Geometry: final body of the model. Coordinates: model frame, mm. Give positions to 0.01 mm unless a question says otherwise; leave off trailing zeros. Order: outer loops, then holes, each group sorted by start corner. A loop starts at its lowest first (then second) coordinate and runs counter-clockwise, first axis right, second up. Notation, with made-up numbers: M 54,88 L 71,88 A19 ccw 71,94 Z; hole C 14.5,-2 d3. An arc over 180 degrees is marked long. Use CSV: the item, a comma, the result in double quotes.
```python
from build123d import *

# Parameters (mm, degrees)
SKETCH1_W           = 224.4
SKETCH1_H           = 224.4
SKETCH1_R           = 1.5
BOSS_EXTRUDE1_DEPTH = 3
FILLET1_R           = 5
SKETCH2_R           = 1
CUT_EXTRUDE1_DEPTH  = 4
SKETCH4_R           = 4.9
CUT_EXTRUDE2_DEPTH  = 4


with BuildPart() as part:
    # Sketch1 → Boss-Extrude1 (new body)
    with BuildSketch(Plane(origin=(0, 0, 0), x_dir=(1, 0, 0), z_dir=(0, 1, 0))):
        with Locations((112.2, 112.2)):
            Rectangle(SKETCH1_W, SKETCH1_H)
        with Locations((213.9, 10.5)):
            Circle(SKETCH1_R, mode=Mode.SUBTRACT)
        with Locations((213.9, 213.9)):
            Circle(SKETCH1_R, mode=Mode.SUBTRACT)
        with Locations((10.5, 10.5)):
            Circle(SKETCH1_R, mode=Mode.SUBTRACT)
        with Locations((10.5, 213.9)):
            Circle(SKETCH1_R, mode=Mode.SUBTRACT)
    extrude(amount=BOSS_EXTRUDE1_DEPTH)

    # Fillet1
    fillet1_edges = [part.edges().sort_by_distance(p)[0] for p in [
        (0, 1.5, -224.4),
        (224.4, 1.5, -224.4),
        (224.4, 1.5, 0),
        (0, 1.5, 0),
    ]]
    fillet(fillet1_edges, radius=FILLET1_R)

    # Sketch2 → Cut-Extrude1 (cut, through all)
    with BuildSketch(Plane(origin=(0, 3, 0), x_dir=(1, 0, 0), z_dir=(0, 1, 0))):
        with Locations((117.180175368, 112.100128542)):
            Circle(SKETCH2_R)
        with Locations((122.180175368, 112.100128542)):
            Circle(SKETCH2_R)
        with Locations((127.180175368, 112.100128542)):
            Circle(SKETCH2_R)
        with Locations((114.680175368, 107.770001523)):
            Circle(SKETCH2_R)
        with Locations((109.680175368, 107.770001523)):
            Circle(SKETCH2_R)
        with Locations((107.180175368, 112.100128542)):
            Circle(SKETCH2_R)
        with Locations((109.680175368, 116.430255561)):
            Circle(SKETCH2_R)
        with Locations((114.680175368, 116.430255561)):
            Circle(SKETCH2_R)
        with Locations((120.840429406, 107.100128542)):
            Circle(SKETCH2_R)
        with Locations((117.180175368, 103.439874505)):
            Circle(SKETCH2_R)
        with Locations((112.180175368, 102.100128542)):
            Circle(SKETCH2_R)
        with Locations((107.180175368, 103.439874505)):
            Circle(SKETCH2_R)
        with Locations((103.51992133, 107.100128542)):
            Circle(SKETCH2_R)
        with Locations((102.180175368, 112.100128542)):
            Circle(SKETCH2_R)
        with Locations((103.51992133, 117.100128542)):
            Circle(SKETCH2_R)
        with Locations((107.180175368, 120.76038258)):
            Circle(SKETCH2_R)
        with Locations((112.180175368, 122.100128542)):
            Circle(SKETCH2_R)
        with Locations((117.180175368, 120.76038258)):
            Circle(SKETCH2_R)
        with Locations((120.840429406, 117.100128542)):
            Circle(SKETCH2_R)
        with Locations((126.669062762, 108.217842866)):
            Circle(SKETCH2_R)
        with Locations((125.170556425, 104.600128542)):
            Circle(SKETCH2_R)
        with Locations((122.786777086, 101.493526825)):
            Circle(SKETCH2_R)
        with Locations((119.680175368, 99.109747486)):
            Circle(SKETCH2_R)
        with Locations((116.062461045, 97.611241148)):
            Circle(SKETCH2_R)
        with Locations((112.180175368, 97.100128542)):
            Circle(SKETCH2_R)
        with Locations((108.297889692, 97.611241148)):
            Circle(SKETCH2_R)
        with Locations((104.680175368, 99.109747486)):
            Circle(SKETCH2_R)
        with Locations((101.57357365, 101.493526825)):
            Circle(SKETCH2_R)
        with Locations((99.189794311, 104.600128542)):
            Circle(SKETCH2_R)
        with Locations((97.691287974, 108.217842866)):
            Circle(SKETCH2_R)
        with Locations((97.180175368, 112.100128542)):
            Circle(SKETCH2_R)
        with Locations((97.691287974, 115.982414219)):
            Circle(SKETCH2_R)
        with Locations((99.189794311, 119.600128542)):
            Circle(SKETCH2_R)
        with Locations((101.57357365, 122.70673026)):
            Circle(SKETCH2_R)
        with Locations((104.680175368, 125.090509599)):
            Circle(SKETCH2_R)
        with Locations((108.297889692, 126.589015937)):
            Circle(SKETCH2_R)
        with Locations((112.180175368, 127.100128542)):
            Circle(SKETCH2_R)
        with Locations((116.062461045, 126.589015937)):
            Circle(SKETCH2_R)
        with Locations((119.680175368, 125.090509599)):
            Circle(SKETCH2_R)
        with Locations((122.786777086, 122.70673026)):
            Circle(SKETCH2_R)
        with Locations((125.170556425, 119.600128542)):
            Circle(SKETCH2_R)
        with Locations((126.669062762, 115.982414219)):
            Circle(SKETCH2_R)
    extrude(amount=-CUT_EXTRUDE1_DEPTH, mode=Mode.SUBTRACT)

    # Sketch4 → Cut-Extrude2 (cut, through all)
    with BuildSketch(Plane(origin=(0, 3, 0), x_dir=(1, 0, 0), z_dir=(0, 1, 0))):
        with Locations((112.2, 157.2)):
            Circle(SKETCH4_R)
        with Locations((157.2, 112.2)):
            Circle(SKETCH4_R)
        with Locations((112.2, 67.2)):
            Circle(SKETCH4_R)
        with Locations((67.2, 112.2)):
            Circle(SKETCH4_R)
    extrude(amount=-CUT_EXTRUDE2_DEPTH, mode=Mode.SUBTRACT)


solid = part.part
```
1. Section A-A, the plane z = -157.2. Return the cut outline in (x, y).
Answer:
outline,"M 0,0 L 107.3,0 L 107.3,3 L 0,3 Z; M 117.1,0 L 224.4,0 L 224.4,3 L 117.1,3 Z"
2. Pull-direction query (X, two-part tool) for faces 1 (the face through (111, 3, -114)), 2 (the face through (1.43, 1.52, -222.9)), 3 (the face through (69.834, 1.521, -116.332)); classes: +X half, -X half, draft (parallel to the pull), parting line (faces both ways), or undercut.
Answer:
face 1,"draft"
face 2,"-X half"
face 3,"undercut"
3. Pin query (flat end, axial travel): pin 1 Ø3 at (x, z) = (117.18, -120.76) entering from -Y. Return the tip coordinate at first contact, or that it passes through.
Answer:
pin 1,"y = 0"
4. Section B-B, the plane x = 66. Return the cut outline in (y, z), plus the area to 3 significant figures.
Answer:
outline,"M 0,-224.4 L 3,-224.4 L 3,-116.95 L 0,-116.95 Z; M 0,-107.45 L 3,-107.45 L 3,0 L 0,0 Z"
area,"645 mm2"
5. Line query: line 1 (Z direction, x = 157.2, y = 1.45); line 2 (Z direction, x = 159.5, y = 0.25); line 3 (Z direction, x = 108.5, y = 0.6). Output: solid intervals per line, ascending.
Answer:
line 1,"-224.4 to -117.1, -107.3 to 0"
line 2,"-224.4 to -116.53, -107.87 to 0"
line 3,"-224.4 to -160.41, -153.99 to -127.57, -125.61 to -98.59, -96.63 to -70.41, -63.99 to 0"
